from build123d import *

# Parameters (mm, degrees)
BOSS_EXTRUDE1_DEPTH = 507.8


with BuildPart() as part:
    # Sketch2 → Boss-Extrude1 (new body)
    with BuildSketch(Plane(origin=(0, 0, 0), x_dir=(0, 0, -1), z_dir=(1, 0, 0))):
        with BuildLine():
            Line((6, -20.036364033), (10.669721768, -20.036364033))
            Line((10.669721768, -20.036364033), (10.669721768, -24.036364033))
            Line((10.669721768, -24.036364033), (-10.669721768, -24.036364033))
            Line((-10.669721768, -24.036364033), (-10.669721768, -20.036364033))
            Line((-10.669721768, -20.036364033), (-6, -20.036364033))
            Line((-6, -20.036364033), (-6, -1.636364033))
            ThreePointArc((-6, -1.636364033), (0, 4.363635967), (6, -1.636364033))
            Line((6, -1.636364033), (6, -20.036364033))
        make_face()
    extrude(amount=BOSS_EXTRUDE1_DEPTH)


solid = part.part
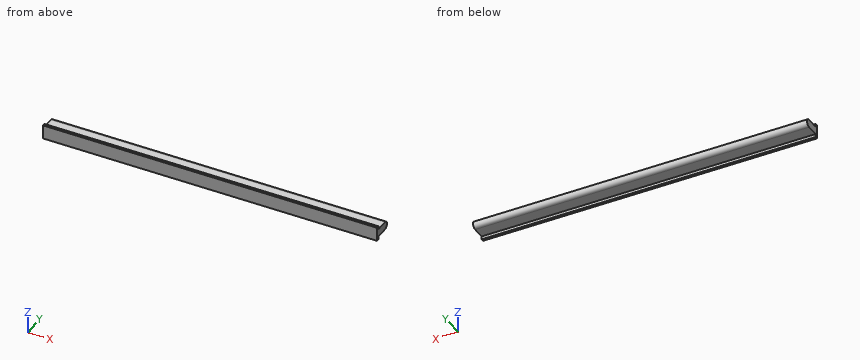
Verification items for the finished model (mm, model axes). Coordinates: 2 decimals unless noted, no trailing zeros. Loops run counter-clockwise (first coordinate to the right, second up) from the corner with the lowest first, then second, coordinate; pieces in that order, holes last. Notation, with made-up numbers: (23.25, 27.25) -> (80.25, 27.25) arc R12 cw to (80.25, 34.25) -> close; hole circle Ø10 at (4.5, -29). An arc over 180 degrees is marked (long way). Answer as CSV lines item,"result".
1) Cross-section at A-A, the plane x = 177. Record the cut outline in (y, z), then the cut area to 3 significant figures.
Found:
outline,"(-24.04, -10.67) -> (-20.04, -10.67) -> (-20.04, -6) -> (-1.64, -6) arc R6 ccw to (-1.64, 6) -> (-20.04, 6) -> (-20.04, 10.67) -> (-24.04, 10.67) -> close"
area,"363 mm2"
2) Depth check by flat-ended pin: pin 1 (5 mm diameter, centred on x = 391, y = -13, fed in from -Z); pin 2 (5 mm diameter, centred on x = 347, z = -7.5, fed in from +Y); pin 3 (5 mm diameter, centred on x = 186, z = 8, fed in from +Y). Enter the tip coordinate at first touch or a pass-through.
Found:
pin 1,"stops at z = -6"
pin 2,"stops at y = 1.68"
pin 3,"stops at y = 0.76"
3) Cross-section at B-B, the plane y = -8.5. Record the cut outline in (x, z), then the cut area to 3 significant figures.
Found:
outline,"(0, -6) -> (507.8, -6) -> (507.8, 6) -> (0, 6) -> close"
area,"6,090 mm2"
4) Thickness scan on L1, parallel to Z at x = 337.5, y = -3.25; L2, parallel to Y at x = 429, z = -7; L3, parallel to Y at x = 38, z = 0.75. Record the ranges inside material, lowest first. Write a range as from..to.
Found:
L1,"z = -6..6"
L2,"y = -24.04..-20.04"
L3,"y = -24.04..4.32"
